Build history of the part. All positions in model axes, mm. Face numbers are marked on the shaded views. A direction names the side the tool comes from. Round coordinates to 2 decimals unless told otherwise and drop trailing zeros. Loops run counter-clockwise (first coordinate to the right, second up) from the corner with the lowest first, then second, coordinate; pieces in that order, holes last. Notation, with made-up numbers: (22, 74.25) - (56, 74.25) arc R21 cw to (56, 81.25) - close; hole circle Ø5 at (10, 63). An arc over 180 degrees is marked (long way). Use one line per item in the form item = value. Start each with the question number.
Q1. 3-axis set-ups, long thin cutter, end or side, ignore diameter. For the marked faces 1 and 2: which of +Z, -Z, +X, -X, +Y, -Y reach the whole face in a straight line?
Q2. Saw through at D-D (z = 23). Give the cut face in (x, y).
Q3. Drill centre lines: line 1 (Z direction, x = -22, y = -7); line 2 (Y direction, x = -45, z = 39.5); line 3 (X direction, y = 10, z = 56). Where is each one in solid material? Low to high.
Q4. Pin check, flat tips, straight feed: pin 1 (12 mm diameter, centred on y = -11, z = 25, fed in from -X); pin 2 (6 mm diameter, centred on x = -26, y = -12.5, fed in from +Z); pin 3 (12 mm diameter, centred on y = 17.5, z = 43, fed in from -X). Stop position of each tip, or through.
Q5. Saw through at C-C (y = 0). Give the cut face in (x, z).
Q6. Saw through at B-B (z = 34.5). Give the cut face in (x, y), then the cut area to 3 significant figures.
Q7. Saw through at A-A (x = -28.5). Give the cut face in (y, z).
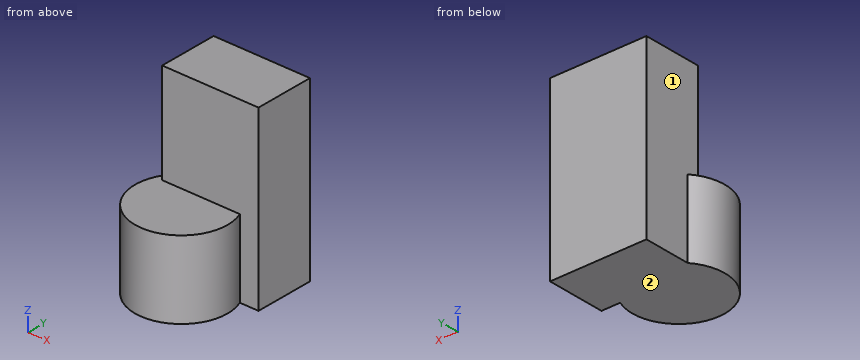
```python
from build123d import *

# Parameters (mm, degrees)
F0_R     = 19.146623
F1_DEPTH = 31.956613
F2_W     = 39.905567
F2_H     = 24.400435
F3_DEPTH = 73.309049


with BuildPart() as f1:
    # F0 (on Top) → F1 (new body)
    with BuildSketch(Plane.XY):
        with Locations((-36.225423, 0)):
            Circle(F0_R)
    extrude(amount=F1_DEPTH)

    # F2 (on Top) → F3 (join)
    with BuildSketch(Plane.XY):
        with Locations((-30.850997, 19.793321)):
            Rectangle(F2_W, F2_H)
    extrude(amount=F3_DEPTH)


solid = f1.part
```
Report:
q1.face_1 = +Z, -X, +Y
q1.face_2 = -Z, +X, -X, +Y, -Y
q2.outline = (-50.8, 12.41) arc R19.15 ccw (long way) to (-18.65, 7.59) - (-10.9, 7.59) - (-10.9, 31.99) - (-50.8, 31.99) - close
q3.line_1 = 0 to 31.96
q3.line_2 = 7.59 to 31.99
q3.line_3 = -50.8 to -10.9
q4.pin_1 = -54.71
q4.pin_2 = 31.96
q4.pin_3 = -50.8
q5.outline = (-55.37, 0) - (-17.08, 0) - (-17.08, 31.96) - (-55.37, 31.96) - close
q6.outline = (-50.8, 7.59) - (-10.9, 7.59) - (-10.9, 31.99) - (-50.8, 31.99) - close
q6.area = 974 mm²
q7.outline = (-17.52, 0) - (31.99, 0) - (31.99, 73.31) - (7.59, 73.31) - (7.59, 31.96) - (-17.52, 31.96) - close
